Design review of the part built by this model. Coordinates are the model's own, in mm. A direction names the side the tool comes from. Coordinates: 2 decimals unless noted, no trailing zeros. Order: outer loops, then holes, each group sorted by start corner. A loop starts at its lowest first (then second) coordinate and runs counter-clockwise, first axis right, second up. Notation, with made-up numbers: (37, -4) -> (61, -4) arc R13 ccw to (61, 21) -> close; hole circle Ø3 at (3, 11.5). An arc over 180 degrees is marked (long way). Write item = value, one per line.
```python
from build123d import *

# Parameters (mm, degrees)
F1_DEPTH       = 70
F2_R           = 6
F4_D           = 2.5
F6_D           = 7
F6_CSINK_D     = 12
F6_CSINK_ANGLE = 90


with BuildPart() as f1:
    # F0 (on Front) → F1 (new body)
    with BuildSketch(Plane.XZ):
        with BuildLine():
            Line((-30.1981142707, 3.3), (-30.1981142707, 0))
            Line((-30.1981142707, 0), (8.4236085474, 0))
            ThreePointArc((8.4236085474, 0), (10.9672225435, 0.509841723), (13.117854557, 1.9605976245))
            Line((13.117854557, 1.9605976245), (16.8330399063, 5.7197011877))
            ThreePointArc((16.8330399063, 5.7197011877), (17.9083559131, 6.4450791385), (19.1801629111, 6.7))
            Line((19.1801629111, 6.7), (39.8018857293, 6.7))
            Line((39.8018857293, 6.7), (39.8018857293, 10))
            Line((39.8018857293, 10), (19.1359616287, 10))
            ThreePointArc((19.1359616287, 10), (16.5778868369, 9.4840984015), (14.4197256433, 8.0170464726))
            Line((14.4197256433, 8.0170464726), (10.7725102503, 4.2914767637))
            ThreePointArc((10.7725102503, 4.2914767637), (9.6934296535, 3.5579507992), (8.4143922576, 3.3))
            Line((8.4143922576, 3.3), (-30.1981142707, 3.3))
        make_face()
    extrude(amount=F1_DEPTH)

    # F2
    f2_edges = [f1.edges().sort_by_distance(p)[0] for p in [
        (-30.198114, 0, 1.65),
        (-30.198114, -70, 1.65),
        (39.801886, -70, 8.35),
        (39.801886, 0, 8.35),
    ]]
    fillet(f2_edges, radius=F2_R)

    # F4 (through all)
    with Locations(Plane.XY.offset(10)):
        with Locations((32.4018857293, -12), (32.4018857293, -58)):
            Hole(F4_D / 2)

    # F6 (through all)
    with Locations(Plane.XY.offset(3.3)):
        with Locations((-20.6981142707, -12), (-20.6981142707, -58)):
            CounterSinkHole(F6_D / 2, F6_CSINK_D / 2, counter_sink_angle=F6_CSINK_ANGLE)


solid = f1.part
```
(1) Insertion check: pin 1 (1.5 mm diameter, centred on x = 32.4, y = -58, fed in from +Z); pin 2 (4 mm diameter, centred on x = -19, y = -11, fed in from -Z); pin 3 (6 mm diameter, centred on x = 31, y = -48, fed in from -Z); pin 4 (6 mm diameter, centred on y = -25.5, z = 8.5, fed in from -X). Each pin has a flat end and moves straight along its axis. Give the tip position at first contact, or say it passes through.
Report:
pin_1 = through
pin_2 = 0
pin_3 = 6.7
pin_4 = 11.96
(2) We need section A-A (y = -12). Write out the cut boundary in (x, z), and give its area (3 significant figures).
Report:
outline = (-30.2, 0) -> (-24.2, 0) -> (-24.2, 0.8) -> (-26.7, 3.3) -> (-30.2, 3.3) -> close; (-17.2, 0) -> (8.42, 0) arc R6.6 ccw to (13.12, 1.96) -> (16.83, 5.72) arc R3.3 cw to (19.18, 6.7) -> (31.15, 6.7) -> (31.15, 10) -> (19.14, 10) arc R6.6 ccw to (14.42, 8.02) -> (10.77, 4.29) arc R3.3 cw to (8.41, 3.3) -> (-14.7, 3.3) -> (-17.2, 0.8) -> close; (33.65, 6.7) -> (39.8, 6.7) -> (39.8, 10) -> (33.65, 10) -> close
area = 201 mm²
(3) We need section B-B (y = -19). Write out the cut boundary in (x, z), and give its area (3 significant figures).
Report:
outline = (-30.2, 0) -> (8.42, 0) arc R6.6 ccw to (13.12, 1.96) -> (16.83, 5.72) arc R3.3 cw to (19.18, 6.7) -> (39.8, 6.7) -> (39.8, 10) -> (19.14, 10) arc R6.6 ccw to (14.42, 8.02) -> (10.77, 4.29) arc R3.3 cw to (8.41, 3.3) -> (-30.2, 3.3) -> close
area = 239 mm²
(4) We need section C-C (x = -0.5). Write out the cut boundary in (y, z).
Report:
outline = (-70, 0) -> (0, 0) -> (0, 3.3) -> (-70, 3.3) -> close
(5) We need section D-D (y = -3.5). Write out the cut boundary in (x, z).
Report:
outline = (-29.65, 0) -> (8.42, 0) arc R6.6 ccw to (13.12, 1.96) -> (16.83, 5.72) arc R3.3 cw to (19.18, 6.7) -> (39.26, 6.7) -> (39.26, 10) -> (19.14, 10) arc R6.6 ccw to (14.42, 8.02) -> (10.77, 4.29) arc R3.3 cw to (8.41, 3.3) -> (-29.65, 3.3) -> close
(6) For L1, parallel to Z at x = -11.5, y = -40.5; L2, parallel to X at y = -58, z = 0.55; L3, parallel to Z at x = 24, y = -64, list the stretches that pass through material, from the lowest coordinate up.
Report:
L1 = 0 to 3.3
L2 = -30.2 to -24.2, -17.2 to 11.06
L3 = 6.7 to 10
(7) For faces 1 (the cylindrical face through (31.73, -56.946, 8.327)), 2 (the flat face through (29, -35, 6.7)), 3 (the flat face through (-11, -35, 3.3)), list the 3-axis set-ups (+Z, -Z, +X, -X, +Y, -Y) from which the entire face can be reached by the end or side of a thin tool; tool diameter is ignored.
Report:
face_1 = +Z, -Z
face_2 = -Z, +X, +Y, -Y
face_3 = +Z, -X, +Y, -Y
(8) The part is to be moulded in two halves that separate along X. For faces 4 (the cylindrical face through (17.892, -34.51, 6.438)), 5 (the cylindrical face through (31.21, -11.62, 8.33)), 6 (the flat face through (30, -35, 10)), 7 (the cylindrical face through (-19.939, -15.417, 0.394)), say which applies: released by +X, released by -X, zero draft, split by the parting line, or undercut.
Report:
face_4 = released by +X
face_5 = undercut
face_6 = zero draft
face_7 = undercut
